```python
from build123d import *

# Parameters (mm, degrees)
SKETCH1_W           = 50
SKETCH1_H           = 5
BOSS_EXTRUDE1_DEPTH = 46
SKETCH2_W           = 38
SKETCH2_H           = 28
CUT_EXTRUDE1_DEPTH  = 46


with BuildPart() as part:
    # Sketch1 → Boss-Extrude1 (new body)
    with BuildSketch(Plane.XY):
        with BuildLine():
            ThreePointArc((-10.25, 0), (0, 10.25), (10.25, 0))
            Line((10.25, 0), (10.25, 25))
            Line((10.25, 25), (-10.25, 25))
            Line((-10.25, 25), (-10.25, 0))
        make_face()
        with BuildLine():
            Line((9.2, 0), (10.25, 0))
            ThreePointArc((10.25, 0), (0, 10.25), (-10.25, 0))
            Line((-10.25, 0), (-9.2, 0))
            ThreePointArc((-9.2, 0), (-8.816088231, 0.879772698), (-7.91, 1.196620241))
            ThreePointArc((-7.91, 1.196620241), (-5.656854249, 5.656854249), (-1.196620241, 7.91))
            ThreePointArc((-1.196620241, 7.91), (-0.045031719, 9.199154762), (1.2, 8))
            ThreePointArc((1.2, 8), (1.199154762, 7.954968281), (1.196620241, 7.91))
            ThreePointArc((1.196620241, 7.91), (5.656854249, 5.656854249), (7.91, 1.196620241))
            ThreePointArc((7.91, 1.196620241), (8.816088231, 0.879772698), (9.2, 0))
        make_face()
        with BuildLine():
            ThreePointArc((6.8, 0), (7.120227302, 0.816088231), (7.91, 1.196620241))
            ThreePointArc((7.91, 1.196620241), (5.656854249, 5.656854249), (1.196620241, 7.91))
            ThreePointArc((1.196620241, 7.91), (0, 6.8), (-1.196620241, 7.91))
            ThreePointArc((-1.196620241, 7.91), (-5.656854249, 5.656854249), (-7.91, 1.196620241))
            ThreePointArc((-7.91, 1.196620241), (-7.120227302, 0.816088231), (-6.8, 0))
            Line((-6.8, 0), (-4.4, 0))
            ThreePointArc((-4.4, 0), (0, 4.4), (4.4, 0))
            Line((4.4, 0), (6.8, 0))
        make_face()
        with BuildLine():
            ThreePointArc((-10.25, 0), (0, -10.25), (10.25, 0))
            Line((10.25, 0), (9.2, 0))
            ThreePointArc((9.2, 0), (8.816088231, -0.879772698), (7.91, -1.196620241))
            ThreePointArc((7.91, -1.196620241), (5.656854249, -5.656854249), (1.196620241, -7.91))
            ThreePointArc((1.196620241, -7.91), (1.199154762, -7.954968281), (1.2, -8))
            ThreePointArc((1.2, -8), (-0.045031719, -9.199154762), (-1.196620241, -7.91))
            ThreePointArc((-1.196620241, -7.91), (-5.656854249, -5.656854249), (-7.91, -1.196620241))
            ThreePointArc((-7.91, -1.196620241), (-8.816088231, -0.879772698), (-9.2, 0))
            Line((-9.2, 0), (-10.25, 0))
        make_face()
        with BuildLine():
            ThreePointArc((1.196620241, -7.91), (5.656854249, -5.656854249), (7.91, -1.196620241))
            ThreePointArc((7.91, -1.196620241), (7.120227302, -0.816088231), (6.8, 0))
            Line((6.8, 0), (4.4, 0))
            ThreePointArc((4.4, 0), (0, -4.4), (-4.4, 0))
            Line((-4.4, 0), (-6.8, 0))
            ThreePointArc((-6.8, 0), (-7.120227302, -0.816088231), (-7.91, -1.196620241))
            ThreePointArc((-7.91, -1.196620241), (-5.656854249, -5.656854249), (-1.196620241, -7.91))
            ThreePointArc((-1.196620241, -7.91), (0, -6.8), (1.196620241, -7.91))
        make_face()
        with Locations((14.75, 27.5)):
            Rectangle(SKETCH1_W, SKETCH1_H)
    extrude(amount=-BOSS_EXTRUDE1_DEPTH)

    # Sketch2 → Cut-Extrude1 (cut)
    with BuildSketch(Plane.ZY.offset(10.25)):
        with Locations((-23, 3.75)):
            Rectangle(SKETCH2_W, SKETCH2_H)
    extrude(amount=-CUT_EXTRUDE1_DEPTH, mode=Mode.SUBTRACT)


solid = part.part
```
CAD build for the part. Positions are in the model's coordinates, mm. A direction names the side the tool comes from. Give positions to 0.01 mm unless a question says otherwise; leave off trailing zeros. Write each loop counter-clockwise with the first axis right and the second up, starting at its lowest first coordinate (ties: lowest second). Pieces come first, ordered by that corner, then holes. Notation, with made-up numbers: M -34.5,84.25 L -19.5,84.25 A26 ccw -19.5,122.25 Z; hole C -0.75,50 d10. An arc over 180 degrees is marked long. Return JSON: item names as keys, results as strings. Group by question number.
(1) Band-saw the part on D-D (x = 17.5). Give the cut face in (y, z), and give its area (3 significant figures).
(2) Band-saw the part on B-B (z = -38). Give the cut face in (x, y), and give its area (3 significant figures).
(3) Drill centre lines: L1, parallel to X at y = 0, z = -43; L2, parallel to Z at x = -2, y = 15; L3, parallel to Y at x = 6, z = -28.5. Where is each one in solid material? Low to high. Write a range as [from, to].
(4) Flat gauge pins, fed straight in: pin 1 Ø8 at (x, y) = (0, 0) entering from -Z; pin 2 Ø12 at (y, z) = (16, -20.5) entering from +X; pin 3 Ø10 at (x, z) = (21.5, -20) entering from -Y. Where does each tip first touch, or does it go through?
(5) Band-saw the part on C-C (y = 20). Give the cut face in (x, z).
(6) Mould opens along Z. For faces 1 (the face through (39.75, 27, -23)), 2 (the face through (-2, 7, -4)), 3 (the face through (3, 15, 0)) say: pulls with the +Z half, pulls with the -Z half, needs draft (parallel to the pull), parting line crosses it, or undercut.
(7) Band-saw the part on A-A (x = 0). State how many separate pieces and enclosed holes the cut face has, and give its area (3 significant figures).
(8) 3-axis set-ups, long thin cutter, end or side, ignore diameter. For faces 4 (the face through (-2, 7, -42)), 5 (the face through (25, 25, -23)), 6 (the face through (-0.225, -10.248, -1.972)): which of +Z, -Z, +X, -X, +Y, -Y reach the whole face in a straight line?
Entries:
{
 "1": {"outline": "M 25,-46 L 30,-46 L 30,0 L 25,0 Z", "area": "230 mm^2"},
 "2": {"outline": "M -10.25,17.75 L 10.25,17.75 L 10.25,25 L 39.75,25 L 39.75,30 L -10.25,30 Z", "area": "399 mm^2"},
 "3": {"L1": "x = [-10.25, -9.2], [-6.8, -4.4], [4.4, 6.8], [9.2, 10.25]", "L2": "z = [-46, -42], [-4, 0]", "L3": "y = [17.75, 30]"},
 "4": {"pin 1": "passes through", "pin 2": "stops at x = 10.25", "pin 3": "stops at y = 25"},
 "5": {"outline": "M -10.25,-46 L 10.25,-46 L 10.25,0 L -10.25,0 Z"},
 "6": {"face 1": "needs draft", "face 2": "undercut", "face 3": "pulls with the +Z half"},
 "7": {"separate pieces": "7", "enclosed holes": "0", "area": "679 mm^2"},
 "8": {"face 4": "+X, -X, -Y", "face 5": "+Z, -Z, +X, -Y", "face 6": "+Z, -Z, -Y"}
}
